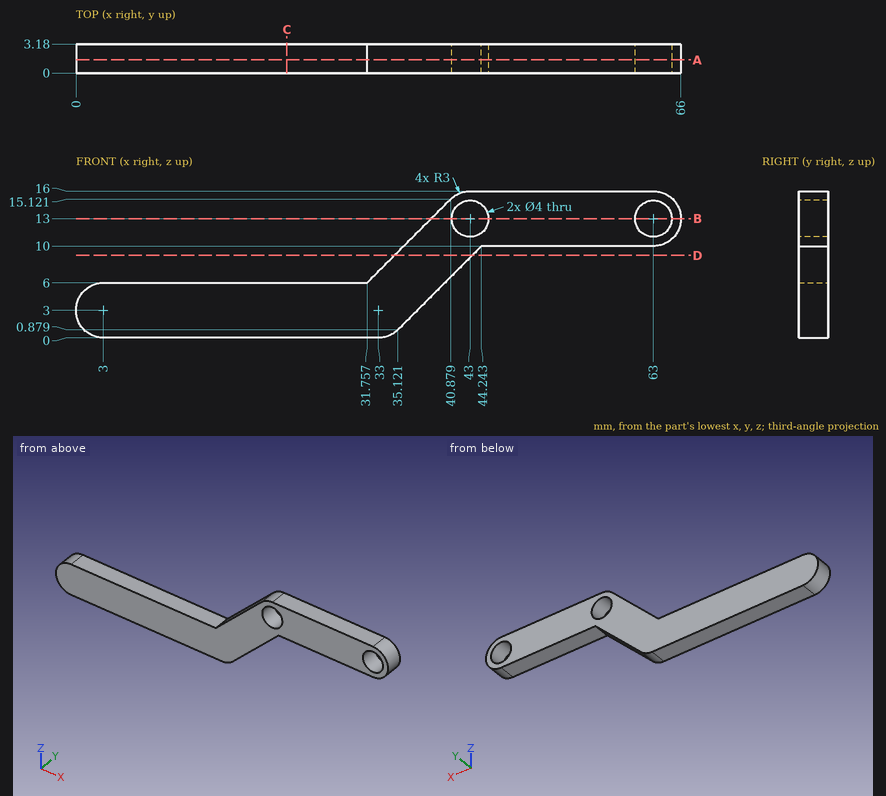
Design review of the part shown in the three views and the two pictorial views. Dimensions are in mm from the part's minimum x, y and z. Give positions to 0.01 mm unless a question says otherwise; leave off trailing zeros. Loops run counter-clockwise (first coordinate to the right, second up) from the corner with the lowest first, then second, coordinate; pieces in that order, holes last. Notation, with made-up numbers: M 11,-38 L 54,-38 A19 ccw 54,-18 Z; hole C 78,31 d10. An arc over 180 degrees is marked long. Answer as a JSON object with one key per item and string values. Group by question number.
Q1. Insertion check: P1, Ø1, axis at x = 18.5, y = 1, coming from the +Z side; P2, Ø2.5, axis at x = 43, z = 13, coming from the +Y side. Each pin has a flat end and moves straight along its axis. Give the tip position at first contact, or say it passes through.
Q2. For probe 1 along Z at (x, y) = (63, 1.45); probe 2 along X at (y, z) = (1.95, 11.75) (1 decimal); probe 3 along Z at (x, y) = (49, 2.35), list the stretches that pass through material, from the lowest coordinate up. Write a range as [from, to].
Q3. Add section D-D on z = 9. Give the boundary of the cut face in (x, y).
Q4. Add section A-A on y = 1.45. Give the boundary of the cut face in (x, z).
Q5. Add section C-C on x = 23. Give the boundary of the cut face in (y, z), and give its area (3 significant figures).
Q6. Add section B-B on z = 13. Give the boundary of the cut face in (x, y).
Checked values:
{
 "1": {"P1": "z = 6", "P2": "through"},
 "2": {"probe 1": "[10, 11], [15, 16]", "probe 2": "[37.5, 41.4], [44.6, 61.4], [64.6, 65.7]", "probe 3": "[10, 16]"},
 "3": {"outline": "M 34.76,0 L 43.24,0 L 43.24,3.18 L 34.76,3.18 Z"},
 "4": {"outline": "M 3,0 L 33,0 A3 ccw 35.12,0.88 L 44.24,10 L 63,10 A3 ccw 63,16 L 43,16 A3 ccw 40.88,15.12 L 31.76,6 L 3,6 A3 ccw Z; hole C 43,13 d4; hole C 63,13 d4"},
 "5": {"outline": "M 0,0 L 3.18,0 L 3.18,6 L 0,6 Z", "area": "19.1 mm²"},
 "6": {"outline": "M 38.76,0 L 41,0 L 41,3.18 L 38.76,3.18 Z; M 45,0 L 61,0 L 61,3.18 L 45,3.18 Z; M 65,0 L 66,0 L 66,3.18 L 65,3.18 Z"}
}
